```python
from build123d import *

# Parameters (mm, degrees)
SKETCH3_W               = 31.75
SKETCH3_H               = 73.557500078
SKETCH3_R               = 2.200000045
BOSS_EXTRUDE1_DEPTH     = 6.35
SKETCH5_W               = 31.75
SKETCH5_H               = 6.35
BOSS_EXTRUDE2_DEPTH     = 50.8
FILLET1_R               = 9.525
SKETCH6_R               = 1.777000002
CUT_EXTRUDE1_DEPTH      = 74.557500078
CUT_EXTRUDE1_DEPTH_BACK = 7.35
CUT_EXTRUDE2_DEPTH      = 51.8
SKETCH8_R               = 3.499999985
CUT_EXTRUDE3_DEPTH      = 70.85


with BuildPart() as part:
    # Sketch3 → Boss-Extrude1 (new body)
    with BuildSketch(Plane(origin=(0, 0, 0), x_dir=(0, 0, -1), z_dir=(1, 0, 0))):
        with Locations((15.875, 36.778750039)):
            Rectangle(SKETCH3_W, SKETCH3_H)
        with Locations((10.874999967, 15.285000037)):
            Circle(SKETCH3_R, mode=Mode.SUBTRACT)
        with Locations((20.875000033, 15.285000037)):
            Circle(SKETCH3_R, mode=Mode.SUBTRACT)
        with Locations((10.874999967, 63.885000119)):
            Circle(SKETCH3_R, mode=Mode.SUBTRACT)
        with Locations((20.875000033, 63.885000119)):
            Circle(SKETCH3_R, mode=Mode.SUBTRACT)
        Polygon((5.748000061, 60.857500078), (14.875, 60.857500078), (14.875, 67.461500078), (16.875, 67.461500078), (16.875, 60.857500078), (26.001999939, 60.857500078), (26.001999939, 18.312500078), (16.875, 18.312500078), (16.875, 11.708500078), (14.875, 11.708500078), (14.875, 18.312500078), (5.748000061, 18.312500078), align=None, mode=Mode.SUBTRACT)
    extrude(amount=BOSS_EXTRUDE1_DEPTH)

    # Sketch5 → Boss-Extrude2 (add)
    with BuildSketch(Plane(origin=(6.35, 0, 0), x_dir=(0, 0, -1), z_dir=(1, 0, 0))):
        with Locations((15.875, -3.175)):
            Rectangle(SKETCH5_W, SKETCH5_H)
    extrude(amount=-BOSS_EXTRUDE2_DEPTH)

    # Fillet1
    fillet1_edges = [part.edges().sort_by_distance(p)[0] for p in [
        (0, 0, -15.875),
    ]]
    fillet(fillet1_edges, radius=FILLET1_R)

    # Sketch6 → Cut-Extrude1 (cut, two sides)
    with BuildSketch(Plane(origin=(0, 0, 0), x_dir=(1, 0, 0), z_dir=(0, 1, 0))) as cut_extrude1_sk:
        with Locations((-6.35, 6.35)):
            Circle(SKETCH6_R)
        with Locations((-38.1, 15.875)):
            Circle(SKETCH6_R)
        with Locations((-6.35, 25.4)):
            Circle(SKETCH6_R)
    extrude(amount=CUT_EXTRUDE1_DEPTH, mode=Mode.SUBTRACT)
    extrude(cut_extrude1_sk.sketch, amount=-CUT_EXTRUDE1_DEPTH_BACK, mode=Mode.SUBTRACT)

    # Sketch7 → Cut-Extrude2 (cut, through all)
    with BuildSketch(Plane(origin=(6.35, 0, 0), x_dir=(0, 0, -1), z_dir=(1, 0, 0))):
        with BuildLine():
            Line((0, 66.918512437), (0, 82.748877538))
            Line((0, 82.748877538), (31.75, 82.748877538))
            Line((31.75, 82.748877538), (31.75, 66.918512437))
            ThreePointArc((31.75, 66.918512437), (15.875, 69.85), (0, 66.918512437))
        make_face()
    extrude(amount=-CUT_EXTRUDE2_DEPTH, mode=Mode.SUBTRACT)

    # Sketch8 → Cut-Extrude3 (cut, through all)
    with BuildSketch(Plane(origin=(0, 0, 0), x_dir=(1, 0, 0), z_dir=(0, 1, 0))):
        with Locations((-6.35, 25.4)):
            Circle(SKETCH8_R)
        with Locations((-6.35, 6.35)):
            Circle(SKETCH8_R)
    extrude(amount=CUT_EXTRUDE3_DEPTH, mode=Mode.SUBTRACT)


solid = part.part
```
Here's how the part is built. I have some questions about the finished solid (model axes, mm). A direction names the side the tool comes from. Give positions to 0.01 mm unless a question says otherwise; leave off trailing zeros. Order: outer loops, then holes, each group sorted by start corner. A loop starts at its lowest first (then second) coordinate and runs counter-clockwise, first axis right, second up. Notation, with made-up numbers: (76.5, 57) -> (90.5, 57) arc R11 ccw to (90.5, 62) -> close; hole circle Ø8 at (33, 25). An arc over 180 degrees is marked (long way). Use CSV: the item, a comma, the result in double quotes. Start each with the question number.
Item 1: If I drill on probe 1 along Z at (x, y) = (-6.35, -4); probe 2 along Z at (x, y) = (3.5, 27); probe 3 along X at (y, z) = (11, -1.5), over which ranges is the centre line in solid material (lowest first)? Write a range as [from, to].
Item 2: Suppose I cut it at B-B (x = -38.1). List the corners of the cut face in (y, z) for me, and give its area (3 significant figures).
Item 3: Suppose I cut it at D-D (x = -6.35). List the corners of the cut face in (y, z) for me, and give its area (3 significant figures).
Item 4: I'm going to push flat-ended pins straight in: P1, Ø3.5, axis at y = 63.885, z = -10.875, coming from the +X side; P2, Ø5.5, axis at x = -38.1, z = -15.875, coming from the +Y side; P3, Ø1, axis at y = 20, z = -3.5, coming from the -X side; P4, Ø3, axis at x = 3.5, z = -22.5, coming from the +Y side. Where does each tip first touch, or does it pass through?
Item 5: Suppose I cut it at C-C (z = -21). Give the number of separate pieces and of enclosed holes in the cut face, and give its area (3 significant figures).
Item 6: On a 3-axis mill with a long thin cutter (end or side, diameter ignored), from which of +Z, -Z, +X, -X, +Y, -Y can I reach the whole of each face in a straight line? I mean faces 1 (the flat face through (-44.45, -3, -16)), 2 (the flat face through (3, 11.709, -16)). Say none if no direction works.
Item 7: Suppose I cut it at A-A (y = 57.5). List the corners of the cut face in (x, z) for me.
Item 8: Thinking about a two-plate mould opening in Z: for faces 3 (the flat face through (4, 17, 0)), 4 (the cylindrical face through (-2.853, 1.043, -25.267)), 5 (the cylindrical face through (3.22, 69.85, -16.1)), which applies, pulls with the +Z half, pulls with the -Z half, needs draft (parallel to the pull), parting line crosses it, or undercut?
Answer block:
1,probe 1,"z = [-31.75, -27.18], [-23.62, -8.13], [-4.57, 0]"
1,probe 2,"z = [-31.75, -26], [-5.75, 0]"
1,probe 3,"x = [0, 6.35]"
2,outline,"(-6.35, -31.75) -> (0, -31.75) -> (0, -17.65) -> (-6.35, -17.65) -> close; (-6.35, -14.1) -> (0, -14.1) -> (0, 0) -> (-6.35, 0) -> close"
2,area,"179 mm^2"
3,outline,"(-6.35, -31.75) -> (0.54, -31.75) -> (0.54, -28.9) -> (0, -28.9) -> (0, -27.18) -> (-6.35, -27.18) -> close; (-6.35, -23.62) -> (0, -23.62) -> (0, -21.9) -> (0.54, -21.9) -> (0.54, -9.85) -> (0, -9.85) -> (0, -8.13) -> (-6.35, -8.13) -> close; (-6.35, -4.57) -> (0, -4.57) -> (0, -2.85) -> (0.54, -2.85) -> (0.54, 0) -> (-6.35, 0) -> close"
3,area,"166 mm^2"
4,P1,"passes through"
4,P2,"stops at y = 0"
4,P3,"stops at x = 0"
4,P4,"stops at y = 69.55"
5,separate pieces,"4"
5,enclosed holes,"0"
5,area,"458 mm^2"
6,face 1,"+Z, -Z, -X, +Y, -Y"
6,face 2,"+X, -X"
7,outline,"(0, -31.75) -> (6.35, -31.75) -> (6.35, -26) -> (0, -26) -> close; (0, -5.75) -> (6.35, -5.75) -> (6.35, 0) -> (0, 0) -> close"
8,face 3,"pulls with the +Z half"
8,face 4,"undercut"
8,face 5,"parting line crosses it"
